Here's how the part is built. I have some questions about the finished solid (model axes, mm). A direction names the side the tool comes from. Round coordinates to 2 decimals unless told otherwise and drop trailing zeros. Loops run counter-clockwise (first coordinate to the right, second up) from the corner with the lowest first, then second, coordinate; pieces in that order, holes last. Notation, with made-up numbers: M 69,49.5 L 119,49.5 A32 cw 119,83.5 Z; hole C 16.25,-24.75 d3. An arc over 180 degrees is marked long. Answer as a JSON object with one key per item and string values.
Autodesk Inventor part; units mm, degrees
ref_plane "YZ Plane" through (0, 0, 0) normal (1, 0, 0) x (0, 1, 0)
ref_plane "XZ Plane" through (0, 0, 0) normal (0, 1, 0) x (-1, 0, 0)
ref_plane "XY Plane" through (0, 0, 0) normal (0, 0, 1) x (1, 0, 0)
sketch "Sketch1" plane through (0, 0, 0) normal (0, 1, 0) x (-1, 0, 0)
  circle A0 centre (0, 0) radius 1
  dimension "d0" = 2
extrude "Extrusion1" add sketch "Sketch1" along normal blind 10
sketch "Sketch2" plane through (0, 10, 0) normal (0, 1, 0) x (1, 0, 0)
  circle A0 centre (0, 0) radius 1.5
  dimension "d3" = 3
extrude "Extrusion2" add sketch "Sketch2" along normal blind 1.2
fillet "Fillet1" radius 1 1 edges at (-1.5, 11.2, 0)
chamfer "Chamfer1" distance 0.3 angle 45 1 edges at (1, 0, 0)
thread "Thread1"
properties part number "M2x10 Screw Steel" material "Nylon 6"
Item 1: If I drill on L1, parallel to X at y = 7.75, z = 0.05; L2, parallel to Y at x = -0.3, z = -1.2, over which ranges is the centre line in solid material (lowest first)? Write a range as from..to.
Solution:
{"L1": "x = -1..1", "L2": "y = 10..10.88"}
Item 2: For P1, Ø1.5, axis at x = 1, y = 1.5, coming from the -Z side, with a flat end and sliding along its axis, tell me the tip position at first contact or that it passes through.
Solution:
{"P1": "stops at z = -0.97"}
Item 3: I want a section at A-A on y = 6.25. List the corners of the cut face in (x, z) for me, plus the area to 3 significant figures.
Solution:
{"outline": "C 0,0 d2", "area": "3.14 mm2"}
Item 4: For faces 1 (the face through (0, 0, 0)), 2 (the face through (0, 5, 1)), which set-ups out of +Z, -Z, +X, -X, +Y, -Y let a thin tool reach every point of the face, with its end or its side?
Solution:
{"face 1": "+Z, -Z, +X, -X, -Y", "face 2": "-Y"}
